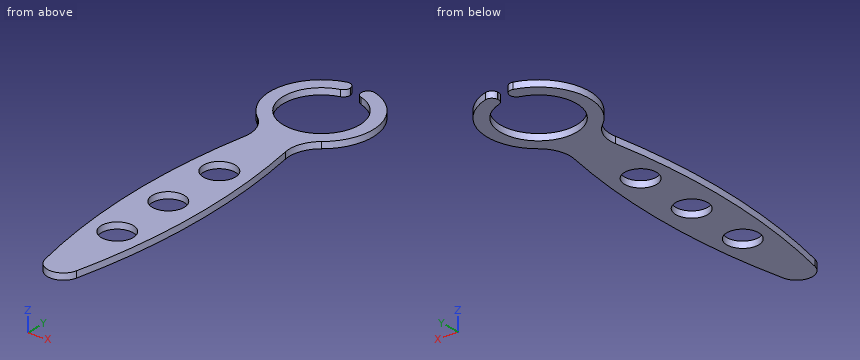
from build123d import *

# Parameters (mm, degrees)
F0_R     = 5
F1_DEPTH = 2
F2_R     = 10
F3_R     = 5
F4_R     = 2


with BuildPart() as f1:
    # F0 (on Top) → F1 (new body)
    with BuildSketch(Plane.XY):
        with BuildLine():
            ThreePointArc((1.553262, 11.798194), (0, -11.9), (-1.553262, 11.798194))
            Line((-1.553262, 11.798194), (-2.088419, 15.863118))
            ThreePointArc((-2.088419, 15.863118), (-15.93017, 1.493216), (-5, -15.198684))
            ThreePointArc((-5, -15.198684), (-9.494839, -67.933061), (0, -120))
            ThreePointArc((0, -120), (9.494839, -67.933061), (5, -15.198684))
            ThreePointArc((5, -15.198684), (15.93017, 1.493216), (2.088419, 15.863118))
            Line((2.088419, 15.863118), (1.553262, 11.798194))
        make_face()
        with Locations((0, -80)):
            Circle(F0_R, mode=Mode.SUBTRACT)
        with Locations((0, -60)):
            Circle(F0_R, mode=Mode.SUBTRACT)
        with Locations((0, -40)):
            Circle(F0_R, mode=Mode.SUBTRACT)
    extrude(amount=F1_DEPTH)

    # F2
    f2_edges = [f1.edges().sort_by_distance(p)[0] for p in [
        (5, -15.198684, 1),
        (-5, -15.198684, 1),
    ]]
    fillet(f2_edges, radius=F2_R)

    # F3
    f3_edges = [f1.edges().sort_by_distance(p)[0] for p in [
        (0, -120, 1),
    ]]
    fillet(f3_edges, radius=F3_R)

    # F4
    f4_edges = [f1.edges().sort_by_distance(p)[0] for p in [
        (-1.553262, 11.798194, 1),
        (1.553262, 11.798194, 1),
        (-2.088419, 15.863118, 1),
        (2.088419, 15.863118, 1),
    ]]
    fillet(f4_edges, radius=F4_R)


solid = f1.part
Input: part model. Units: mm. Frame: model coordinates. Coordinates: 2 decimals unless noted, no trailing zeros. Loops run counter-clockwise (first coordinate to the right, second up) from the corner with the lowest first, then second, coordinate; pieces in that order, holes last. Notation, with made-up numbers: (-38.5, 80.5) -> (-0.5, 80.5) arc R12 cw to (-0.5, 103.5) -> close; hole circle Ø10 at (-8, -18.5). An arc over 180 degrees is marked (long way). Write each question's results on one line, items separated by ' | '. Start each with the question number.
Q1. Pin query (flat end, axial travel): pin 1 (1.5 mm diameter, centred on x = 10.5, y = -53.5, fed in from -Z). Return the tip coordinate at first contact, or that it passes through.
Q2. Section B-B, the plane y = -61.5. Return the cut outline in (x, z).
Q3. Section A-A, the plane y = 0. Return the cut outline in (x, z).
Q4. Ray query, line 1 (Y direction, x = 0, z = 1.55); line 2 (X direction, y = -57.5, z = 1.75); line 3 (X direction, y = -60.5, z = 1.35). Return the intervals inside material, ascending. Write a range as from..to.
Q5. Section C-C, the plane z = 0.4. State how many separate pieces and enclosed holes the cut face has, plus the area to 3 significant figures.
Q6. Section D-D, the plane x = 14. Return the cut outline in (y, z).
Found:
1) pin 1: through
2) outline: (-9.7, 0) -> (-4.77, 0) -> (-4.77, 2) -> (-9.7, 2) -> close; (4.77, 0) -> (9.7, 0) -> (9.7, 2) -> (4.77, 2) -> close
3) outline: (-16, 0) -> (-11.9, 0) -> (-11.9, 2) -> (-16, 2) -> close; (11.9, 0) -> (16, 0) -> (16, 2) -> (11.9, 2) -> close
4) line 1: -106.06..-85, -75..-65, -55..-45, -35..-11.9 | line 2: -9.72..-4.33, 4.33..9.72 | line 3: -9.71..-4.97, 4.97..9.71
5) separate pieces: 1 | enclosed holes: 3 | area: 1,560 mm2
6) outline: (-7.75, 0) -> (7.75, 0) -> (7.75, 2) -> (-7.75, 2) -> close
